```python
from build123d import *

# Parameters (mm, degrees)
F0_R          = 20
F1_DEPTH      = 13
F3_DEPTH      = 25
F3_DEPTH_BACK = 5
F4_R          = 1.5
F5_DEPTH      = 13.001


with BuildPart() as f1:
    # F0 (on Top) → F1 (new body)
    with BuildSketch(Plane.XY):
        Circle(F0_R)
    extrude(amount=F1_DEPTH)

    # F2 (on Right) → F3 (cut, two sides)
    with BuildSketch(Plane.YZ) as f3_sk:
        Polygon((-9, 2), (-9, 0), (9, 0), (9, 2), (10.1, 2), (10.1, 4.1), (-10.1, 4.1), (-10.1, 2), align=None)
    extrude(amount=-F3_DEPTH, mode=Mode.SUBTRACT)
    extrude(f3_sk.sketch, amount=F3_DEPTH_BACK, mode=Mode.SUBTRACT)

    # F4 (on face) → F5 (cut, through all)
    with BuildSketch(Plane.XY.offset(13)):
        with Locations((-9, 0)):
            Circle(F4_R)
        with Locations((9, 0)):
            Circle(F4_R)
    extrude(amount=-F5_DEPTH, mode=Mode.SUBTRACT)


solid = f1.part
```
The model under review builds one solid part; all positions refer to its coordinate system, in mm. A direction names the side the tool comes from. Give positions to 0.01 mm unless a question says otherwise; leave off trailing zeros. Write each loop counter-clockwise with the first axis right and the second up, starting at its lowest first coordinate (ties: lowest second). Pieces come first, ordered by that corner, then holes. Notation, with made-up numbers: M 53,79 L 79,79 A25 ccw 79,94 Z; hole C -7.75,71.25 d10. An arc over 180 degrees is marked long. Answer in a Markdown table with one row per item.
Item 1: Add section D-D on z = 3.5. Give the boundary of the cut face in (x, y).
Check sheet entries:
| item | result |
|---|---|
| outline | M -17.26,-10.1 A20 ccw long -17.26,10.1 L 5,10.1 L 5,-10.1 Z; hole C 9,0 d3 |
Item 2: Tool access review of faces 4 (the face through (-6, -9, 1)), 5 (the face through (0, 0, 13)), 6 (the face through (-6.3, -9.6, 2)): name each direction out of +Z, -Z, +X, -X, +Y, -Y from which nothing blocks a thin tool from reaching the whole face with its end or side.
Check sheet entries:
| item | result |
|---|---|
| face 4 | -Z, -X |
| face 5 | +Z, +X, -X, +Y, -Y |
| face 6 | -X |
Item 3: Add section A-A on y = 0. Give the boundary of the cut face in (x, z).
Check sheet entries:
| item | result |
|---|---|
| outline | M -20,4.1 L -10.5,4.1 L -10.5,13 L -20,13 Z; M -7.5,4.1 L 5,4.1 L 5,0 L 7.5,0 L 7.5,13 L -7.5,13 Z; M 10.5,0 L 20,0 L 20,13 L 10.5,13 Z |
Item 4: Add section C-C on z = 10.25. Give the boundary of the cut face in (x, y), plus the area to 3 significant figures.
Check sheet entries:
| item | result |
|---|---|
| outline | C 0,0 d40; hole C -9,0 d3; hole C 9,0 d3 |
| area | 1,240 mm2 |
Item 5: For P1, Ø0.6, axis at x = -8, z = 2.5, coming from the +Y side; P2, Ø4, axis at x = 16, z = 3.5, coming from the +Y side; P3, Ø1.5, axis at x = -15.5, z = 2.5, coming from the -Y side; P4, Ø12, axis at x = 2, y = 10.5, coming from the -Z side, all flat-tipped, find the tip position at first contact; note any pin that passes through.
Check sheet entries:
| item | result |
|---|---|
| P1 | y = 18.46 |
| P2 | y = 14.28 |
| P3 | y = -13.51 |
| P4 | z = 0 |
Item 6: For line 1 along Z through (x, y) = (-10, 10); line 2 along Y through (x, z) = (9, 10); line 3 along Z through (x, y) = (-15, -5), list the stretches that pass through material, from the lowest coordinate up.
Check sheet entries:
| item | result |
|---|---|
| line 1 | 0 to 2, 4.1 to 13 |
| line 2 | -17.86 to -1.5, 1.5 to 17.86 |
| line 3 | 4.1 to 13 |
Item 7: Add section B-B on x = -9. Give the boundary of the cut face in (y, z), plus the area to 3 significant figures.
Check sheet entries:
| item | result |
|---|---|
| outline | M -17.86,0 L -9,0 L -9,2 L -10.1,2 L -10.1,4.1 L -1.5,4.1 L -1.5,13 L -17.86,13 Z; M 1.5,4.1 L 10.1,4.1 L 10.1,2 L 9,2 L 9,0 L 17.86,0 L 17.86,13 L 1.5,13 Z |
| area | 359 mm2 |
Item 8: Draft analysis for pull direction Z (two halves, no side actions). For faces 1 (the face through (-6, 10.1, 3)), 2 (the face through (-10.5, 0.07, 8.61)), 3 (the face through (9, 5, 0)), state which applies: +Z half, -Z half, draft (parallel to the pull), parting line (faces both ways), or undercut.
Check sheet entries:
| item | result |
|---|---|
| face 1 | undercut |
| face 2 | draft |
| face 3 | -Z half |
